```python
from build123d import *

# Parameters (mm, degrees)
SKETCH1_W          = 38.1
SKETCH1_H          = 38.1
SKETCH1_R          = 12.7254
EXTRUDE1_DEPTH     = 9.525
CUT_EXTRUDE1_DEPTH = 5.5372
HOLE1_D            = 5.5372
HOLE1_DEPTH        = 3.9878


with BuildPart() as part:
    # Sketch1 → Extrude1 (new body)
    with BuildSketch(Plane(origin=(0, 0, 0), x_dir=(1, 0, 0), z_dir=(0, 1, 0))):
        Rectangle(SKETCH1_W, SKETCH1_H)
        with Locations(Location((0, 0, 0), (0, 0, 270))):  # turned: the seam where the file's is
            Circle(SKETCH1_R, mode=Mode.SUBTRACT)
    extrude(amount=EXTRUDE1_DEPTH)

    # Sketch2 → Cut-Extrude1 (cut)
    with BuildSketch(Plane(origin=(0, 9.525, 0), x_dir=(1, 0, 0), z_dir=(0, 1, 0))):
        with BuildLine():
            Line((7.081129237, -19.05), (19.05, -19.05))
            Line((19.05, -19.05), (19.05, -7.081129237))
            ThreePointArc((19.05, -7.081129237), (10.780943879, -10.780943879), (7.081129237, -19.05))
        make_face()
        with BuildLine():
            Line((19.05, 19.05), (19.05, 7.081129237))
            ThreePointArc((19.05, 7.081129237), (10.780943879, 10.780943879), (7.081129237, 19.05))
            Line((7.081129237, 19.05), (19.05, 19.05))
        make_face()
        with BuildLine():
            Line((-7.081129237, 19.05), (-19.05, 19.05))
            Line((-19.05, 19.05), (-19.05, 7.081129237))
            ThreePointArc((-19.05, 7.081129237), (-10.780943879, 10.780943879), (-7.081129237, 19.05))
        make_face()
        with BuildLine():
            Line((-19.05, -19.05), (-19.05, -7.081129237))
            ThreePointArc((-19.05, -7.081129237), (-10.780943879, -10.780943879), (-7.081129237, -19.05))
            Line((-7.081129237, -19.05), (-19.05, -19.05))
        make_face()
    extrude(amount=-CUT_EXTRUDE1_DEPTH, mode=Mode.SUBTRACT)

    # Hole1
    with Locations(Plane(origin=(0, 3.9878, 0), x_dir=(-1, 0, 0), z_dir=(0, 1, 0))):
        with Locations((14.3002, 14.3002), (14.3002, -14.2748), (-14.2748, 14.3002), (-14.2748, -14.2748)):
            Hole(HOLE1_D / 2, depth=HOLE1_DEPTH)

    # Sketch5 → Cut-Revolve1 (revolve, cut)
    with BuildSketch(Plane(origin=(0, 0, 0), x_dir=(0, 0, -1), z_dir=(1, 0, 0)), mode=Mode.PRIVATE) as cut_revolve1_sk:
        Polygon((-13.843, 9.525), (-12.7254, 9.525), (-12.7254, 8.4074), align=None)
        Polygon((-12.7254, 1.1176), (-13.843, 0), (-12.7254, 0), align=None)
    revolve(cut_revolve1_sk.sketch.rotate(Axis((0, 0, 0), (0, 1, 0)), 180), axis=Axis((0, 0, 0), (0, 1, 0)), mode=Mode.SUBTRACT)  # turned: the seam where the file's is


solid = part.part
```
Read the model definition and answer for the solid it produces. Units are mm, in the model's axes. A direction names the side the tool comes from. Give positions to 0.01 mm unless a question says otherwise; leave off trailing zeros. Write each loop counter-clockwise with the first axis right and the second up, starting at its lowest first coordinate (ties: lowest second). Pieces come first, ordered by that corner, then holes. Notation, with made-up numbers: M 70,12.5 L 97,12.5 A29 ccw 97,39.5 Z; hole C 81,79.5 d5. An arc over 180 degrees is marked long. Put each result on its own line as item: value. Start each with the question number.
1. The part is cut by section A-A, the plane z = 0. Give the vertices of the cut face in (x, y) (3 decimals), and give its area (3 significant figures).
2. The part is cut by section D-D, the plane y = 1.75. Give the vertices of the cut face in (x, z).
3. For a pull along X with two mould halves and no side action, classify faces 1 (the cylindrical face through (10.87, 6.8, 10.69)), 2 (the flat face through (0, 4, -19.05)), 3 (the cylindrical face through (16.83, 1.97, -15.34)), 4 (the cylindrical face through (-14.9, 1.966, -16.978)) as released by +X, released by -X, zero draft, split by the parting line, or undercut.
4. Each of these flat-tipped pins is pushed along its axis until it touches: pin 1 Ø9 at (x, z) = (14.27, -14.27) entering from +Y; pin 2 Ø4.5 at (x, z) = (14.27, 14.3) entering from +Y; pin 3 Ø10 at (x, z) = (-8, 7) entering from -Y; pin 4 Ø2 at (x, z) = (7.5, 10) entering from -Y. Where does it stop, or does it pass through?
5. The part is cut by section B-B, the plane x = 0. Give the vertices of the cut face in (y, z) (3 decimals), and give its area (3 significant figures).
6. Consider line 1 along Z through (x, y) = (14.5, 1.75); line 2 along X through (y, z) = (6.75, 0); line 3 along Y through (x, z) = (-12, -12.5). Determine where each line is inside the solid, lowest interval first.
7. The part is cut by section C-C, the plane y = 5.5. Give the vertices of the cut face in (x, z), and give its area (3 significant figures).
8. Which of the six approach directions +Z, -Z, +X, -X, +Y, -Y give full straight-line access (tool end or side, diameter ignored) to faces 5 (the flat face through (12.98, 3.988, 11.65)), 6 (the cylindrical face through (-10.87, 6.8, 10.69)), 7 (the flat face through (-11.8, 3.988, -15.8))?
Final values:
1. outline: M -19.05,0 L -13.843,0 L -12.725,1.118 L -12.725,8.407 L -13.843,9.525 L -19.05,9.525 Z; M 12.725,1.118 L 13.843,0 L 19.05,0 L 19.05,9.525 L 13.843,9.525 L 12.725,8.407 Z
1. area: 118 mm²
2. outline: M -19.05,-19.05 L 19.05,-19.05 L 19.05,19.05 L -19.05,19.05 Z; hole C -14.3,-14.27 d5.54; hole C -14.3,14.3 d5.54; hole C 0,0 d25.45; hole C 14.27,-14.27 d5.54; hole C 14.27,14.3 d5.54
3. face 1: released by +X
3. face 2: zero draft
3. face 3: undercut
3. face 4: undercut
4. pin 1: stops at y = 3.99
4. pin 2: passes through
4. pin 3: stops at y = 0
4. pin 4: stops at y = 0.34
5. outline: M 0,-19.05 L 9.525,-19.05 L 9.525,-13.843 L 8.407,-12.725 L 1.118,-12.725 L 0,-13.843 Z; M 0,13.843 L 1.118,12.725 L 8.407,12.725 L 9.525,13.843 L 9.525,19.05 L 0,19.05 Z
5. area: 118 mm²
6. line 1: z = -19.05 to -17.03, -11.52 to 11.54, 17.06 to 19.05
6. line 2: x = -19.05 to -12.73, 12.73 to 19.05
6. line 3: y = 0 to 3.99
7. outline: M -19.05,-7.08 A12.7 cw -7.08,-19.05 L 7.08,-19.05 A12.7 cw 19.05,-7.08 L 19.05,7.08 A12.7 cw 7.08,19.05 L -7.08,19.05 A12.7 cw -19.05,7.08 Z; hole C 0,0 d25.45
7. area: 506 mm²
8. face 5: +Z, +X, +Y
8. face 6: +Z, -X, +Y
8. face 7: -Z, -X, +Y
